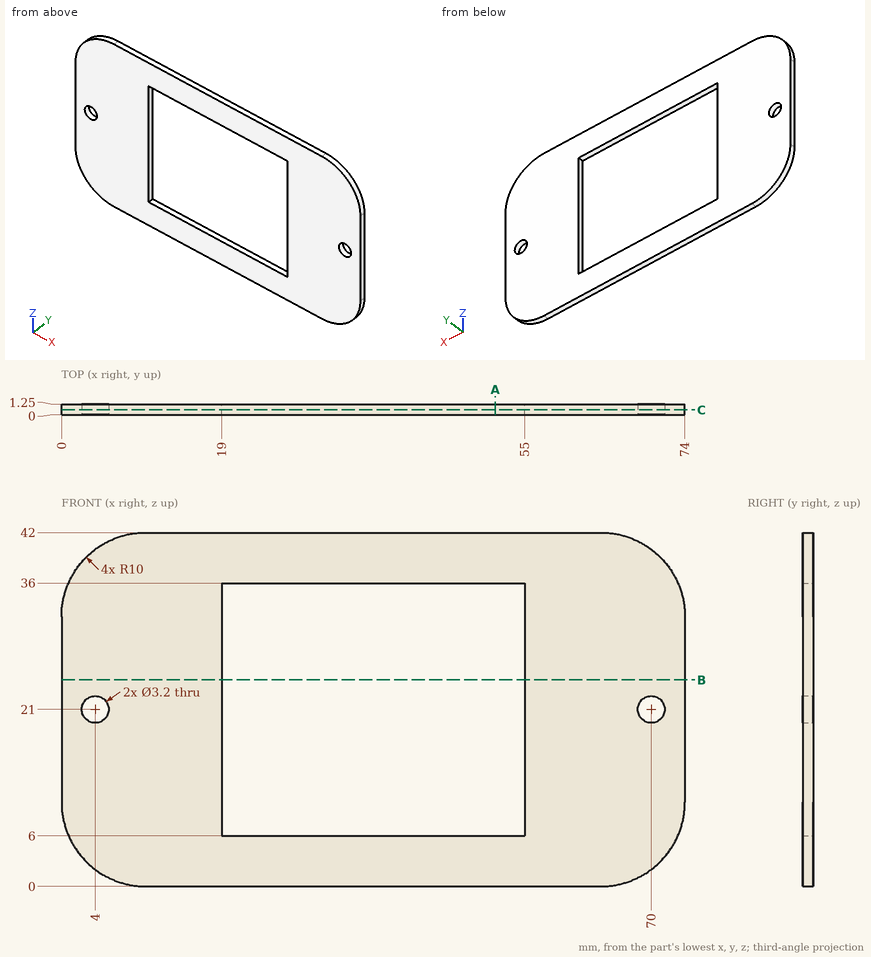
Drawing for the job (mm, zero at the part's lowest x, y, z). Round coordinates to 2 decimals unless told otherwise and drop trailing zeros. Write each loop counter-clockwise with the first axis right and the second up, starting at its lowest first coordinate (ties: lowest second). Pieces come first, ordered by that corner, then holes. Notation, with made-up numbers: M 67,54 L 93,54 A31 cw 93,80 Z; hole C 19.5,-10 d6. An arc over 180 degrees is marked long. One line per question, with ' | ' between items.
1. Cut at C-C on y = 0.55. Write the cut outline in (x, z), and give its area (3 significant figures).
Working result:
outline: M 0,10 A10 ccw 10,0 L 64,0 A10 ccw 74,10 L 74,32 A10 ccw 64,42 L 10,42 A10 ccw 0,32 Z; hole C 4,21 d3.2; hole M 19,6 L 55,6 L 55,36 L 19,36 Z; hole C 70,21 d3.2 | area: 1,930 mm2
2. Probe L1, parallel to X at y = 0.45, z = 21; L2, parallel to Z at x = 26, y = 0.3; L3, parallel to X at y = 0.65, z = 9.5. List the from-to ranges inside material, lowest first. Write a range as from..to.
Working result:
L1: 0..2.4, 5.6..19, 55..68.4, 71.6..74 | L2: 0..6, 36..42 | L3: 0.01..19, 55..73.99
3. Pin check, flat tip, straight feed: pin 1 Ø0.6 at (y, z) = (0.5, 25.5) entering from -X. Stop position of the tip, or through.
Working result:
pin 1: x = 0
4. Cut at A-A on x = 51.5. Write the cut outline in (y, z).
Working result:
outline: M 0,0 L 1.25,0 L 1.25,6 L 0,6 Z; M 0,36 L 1.25,36 L 1.25,42 L 0,42 Z
5. Cut at B-B on z = 24.5. Write the cut outline in (x, y).
Working result:
outline: M 0,0 L 19,0 L 19,1.25 L 0,1.25 Z; M 55,0 L 74,0 L 74,1.25 L 55,1.25 Z
